For this review, take the finished solid that the model builds, in its own axes (mm). Round coordinates to 2 decimals unless told otherwise and drop trailing zeros. Loops run counter-clockwise (first coordinate to the right, second up) from the corner with the lowest first, then second, coordinate; pieces in that order, holes last.
1. Consider section C-C on y = 17. State how many separate pieces and enclosed holes the cut face has, then the cut area to 3 significant figures.
2. Consider section B-B on x = -45.5. State the section outline as (y, z) points.
3. Consider section A-A on x = -15. State the section outline as (y, z) points, then the cut area to 3 significant figures.
4. To check wall thickness, follow line 1 along Y through (x, z) = (-16, 9.5); line 2 along Y through (x, z) = (-145, 9.25); line 3 along Y through (x, z) = (-90, 10.5). State the ranges of each line that lie inside material, in increasing order.
5. Clearance check with flat-ended pins moving along their axes: pin 1 Ø4 at (x, y) = (-110.5, 16) entering from -Z; pin 2 Ø2.5 at (y, z) = (147.5, 12.5) entering from -X; pin 3 Ø3 at (x, y) = (-124, 67.5) entering from +Z. State where each tip first meets the part, or that it passes through.
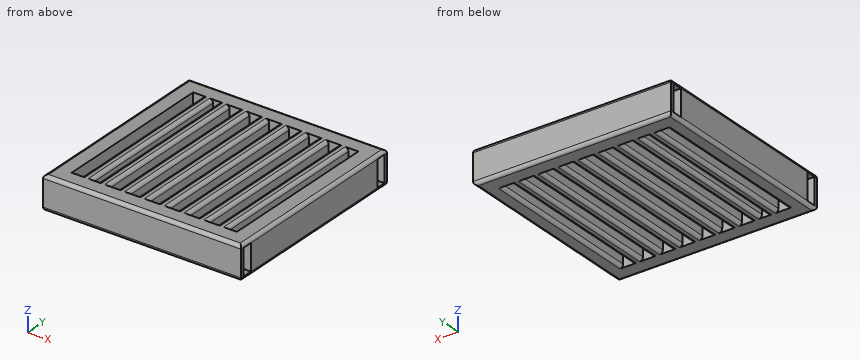
from build123d import *

# Parameters (mm, degrees)
SKETCH1_W           = 152.4
SKETCH1_H           = 152.4
BOSS_EXTRUDE1_DEPTH = 25.4
SKETCH7_W           = 20.32
SKETCH7_H           = 7.62
CUT_EXTRUDE4_DEPTH  = 25.4
SKETCH8_W           = 20.32
SKETCH8_H           = 7.62
CUT_EXTRUDE5_DEPTH  = 25.4
SKETCH9_W           = 7.62
SKETCH9_H           = 127
SKETCH9_W_2         = 5.08
CUT_EXTRUDE6_DEPTH  = 25.4
FILLET3_R           = 2.54
FILLET4_R           = 2.54
FILLET5_DEPTH       = 152.4
FILLET5_START       = -153
FILLET5_2_DEPTH     = 154
FILLET6_R           = 2.54
SKETCH11_W          = 20.32
SKETCH11_H          = 7.62
CUT_EXTRUDE8_DEPTH  = 25.4
SKETCH12_W          = 20.32
SKETCH12_H          = 7.62
CUT_EXTRUDE9_DEPTH  = 25.4


with BuildPart() as part:
    # Sketch1 → Boss-Extrude1 (new body)
    with BuildSketch(Plane.XY):
        with Locations((-76.2, 76.2)):
            Rectangle(SKETCH1_W, SKETCH1_H)
    extrude(amount=BOSS_EXTRUDE1_DEPTH)

    # Sketch7 → Cut-Extrude4 (cut)
    with BuildSketch(Plane(origin=(0, 0, 0), x_dir=(0, 0, -1), z_dir=(1, 0, 0))):
        with Locations((-12.7, 146.05)):
            Rectangle(SKETCH7_W, SKETCH7_H)
    extrude(amount=-CUT_EXTRUDE4_DEPTH, mode=Mode.SUBTRACT)

    # Sketch8 → Cut-Extrude5 (cut)
    with BuildSketch(Plane(origin=(0, 0, 0), x_dir=(0, 0, -1), z_dir=(1, 0, 0))):
        with Locations((-12.7, 6.35)):
            Rectangle(SKETCH8_W, SKETCH8_H)
    extrude(amount=-CUT_EXTRUDE5_DEPTH, mode=Mode.SUBTRACT)

    # Sketch9 → Cut-Extrude6 (cut)
    with BuildSketch(Plane.XY.offset(25.4)):
        with Locations((-135.89, 76.2)):
            Rectangle(SKETCH9_W, SKETCH9_H)
        with Locations((-121.92, 76.2)):
            Rectangle(SKETCH9_W_2, SKETCH9_H)
        with Locations((-107.95, 76.2)):
            Rectangle(SKETCH9_W, SKETCH9_H)
        with Locations((-92.71, 76.2)):
            Rectangle(SKETCH9_W, SKETCH9_H)
        with Locations((-77.47, 76.2)):
            Rectangle(SKETCH9_W, SKETCH9_H)
        with Locations((-62.23, 76.2)):
            Rectangle(SKETCH9_W, SKETCH9_H)
        with Locations((-46.99, 76.2)):
            Rectangle(SKETCH9_W, SKETCH9_H)
        with Locations((-31.75, 76.2)):
            Rectangle(SKETCH9_W, SKETCH9_H)
        with Locations((-16.51, 76.2)):
            Rectangle(SKETCH9_W, SKETCH9_H)
    extrude(amount=-CUT_EXTRUDE6_DEPTH, mode=Mode.SUBTRACT)

    # Fillet3
    fillet3_edges = [part.edges().sort_by_distance(p)[0] for p in [
        (-73.66, 76.2, 25.4),
        (-81.28, 76.2, 25.4),
        (-58.42, 76.2, 25.4),
        (-66.04, 76.2, 25.4),
        (-43.18, 76.2, 25.4),
        (-50.8, 76.2, 25.4),
        (-27.94, 76.2, 25.4),
        (-35.56, 76.2, 25.4),
        (-20.32, 76.2, 25.4),
        (-132.08, 76.2, 25.4),
        (-119.38, 76.2, 25.4),
        (-124.46, 76.2, 25.4),
        (-104.14, 76.2, 25.4),
        (-111.76, 76.2, 25.4),
        (-88.9, 76.2, 25.4),
        (-96.52, 76.2, 25.4),
    ]]
    fillet(fillet3_edges, radius=FILLET3_R)

    # Fillet4
    fillet4_edges = [part.edges().sort_by_distance(p)[0] for p in [
        (-81.28, 76.2, 0),
        (-73.66, 76.2, 0),
        (-66.04, 76.2, 0),
        (-58.42, 76.2, 0),
        (-50.8, 76.2, 0),
        (-43.18, 76.2, 0),
        (-35.56, 76.2, 0),
        (-27.94, 76.2, 0),
        (-20.32, 76.2, 0),
        (-12.7, 76.2, 0),
        (-139.7, 76.2, 0),
        (-132.08, 76.2, 0),
        (-124.46, 76.2, 0),
        (-119.38, 76.2, 0),
        (-111.76, 76.2, 0),
        (-104.14, 76.2, 0),
        (-96.52, 76.2, 0),
        (-88.9, 76.2, 0),
    ]]
    fillet(fillet4_edges, radius=FILLET4_R)

    # Fillet5: read off the stored shape, not the designer's step
    # Fillet5 outline → Fillet5 (cut)
    with BuildSketch(Plane(origin=(0, 0, 0), x_dir=(1, 0, 0), z_dir=(0, 1, 0))):
        with BuildLine():
            Line((-152.4, 0), (-152.4, -2.54))
            ThreePointArc((-152.4, -2.54), (-151.656051224, -0.743948776), (-149.86, 0))
            Line((-149.86, 0), (-152.4, 0))
        make_face()
        with BuildLine():
            Line((0, 0), (-2.54, 0))
            ThreePointArc((-2.54, 0), (-0.743948776, -0.743948776), (0, -2.54))
            Line((0, -2.54), (0, 0))
        make_face()
    extrude(amount=FILLET5_DEPTH, mode=Mode.SUBTRACT)

    # Fillet5 2 outline → Fillet5 2 (cut)
    with BuildSketch(Plane.YZ.offset(FILLET5_START)):
        with BuildLine():
            ThreePointArc((152.4, 2.54), (151.656051224, 0.743948776), (149.86, 0))
            Line((149.86, 0), (152.4, 0))
            Line((152.4, 0), (152.4, 2.54))
        make_face()
        with BuildLine():
            ThreePointArc((2.54, 0), (0.743948776, 0.743948776), (0, 2.54))
            Line((0, 2.54), (0, 0))
            Line((0, 0), (2.54, 0))
        make_face()
    extrude(amount=FILLET5_2_DEPTH, mode=Mode.SUBTRACT)

    # Fillet6
    fillet6_edges = [part.edges().sort_by_distance(p)[0] for p in [
        (-152.4, 76.2, 25.4),
        (-76.2, 0, 25.4),
        (0, 76.2, 25.4),
        (-76.2, 152.4, 25.4),
    ]]
    fillet(fillet6_edges, radius=FILLET6_R - 0.0001)  # a hair under: the kernel refuses the full size

    # Sketch11 → Cut-Extrude8 (cut)
    with BuildSketch(Plane.ZY.offset(152.4)):
        with Locations((12.7, 146.05)):
            Rectangle(SKETCH11_W, SKETCH11_H)
    extrude(amount=-CUT_EXTRUDE8_DEPTH, mode=Mode.SUBTRACT)

    # Sketch12 → Cut-Extrude9 (cut)
    with BuildSketch(Plane.ZY.offset(152.4)):
        with Locations((12.7, 6.35)):
            Rectangle(SKETCH12_W, SKETCH12_H)
    extrude(amount=-CUT_EXTRUDE9_DEPTH, mode=Mode.SUBTRACT)


solid = part.part
Resolved:
1. separate pieces: 10
1. enclosed holes: 0
1. area: 2,140 mm2
2. outline: (0, 2.54) arc R2.54 ccw to (2.54, 0) - (12.7, 0) - (12.7, 25.4) - (2.54, 25.4) arc R2.54 ccw to (0, 22.86) - close; (139.7, 0) - (149.86, 0) arc R2.54 ccw to (152.4, 2.54) - (152.4, 22.86) arc R2.54 ccw to (149.86, 25.4) - (139.7, 25.4) - close
3. outline: (0, 2.54) arc R2.54 ccw to (2.54, 0) - (12.7, 0) - (12.7, 25.4) - (2.54, 25.4) arc R2.54 ccw to (0, 22.86) - close; (139.7, 0) - (149.86, 0) arc R2.54 ccw to (152.4, 2.54) - (152.4, 22.86) arc R2.54 ccw to (149.86, 25.4) - (139.7, 25.4) - close; hole (2.54, 2.54) - (10.16, 2.54) - (10.16, 22.86) - (2.54, 22.86) - close; hole (142.24, 2.54) - (149.86, 2.54) - (149.86, 22.86) - (142.24, 22.86) - close
3. area: 330 mm2
4. line 1: y = 0 to 2.54, 10.16 to 12.7, 139.7 to 142.24, 149.86 to 152.4
4. line 2: y = 0 to 2.54, 10.16 to 142.24, 149.86 to 152.4
4. line 3: y = 0 to 12.7, 139.7 to 152.4
5. pin 1: stops at z = 0.75
5. pin 2: stops at x = -127
5. pin 3: stops at z = 24.91
